Geometry check sheet. Reference: drawing and pictorial views, mm from the part's lowest x, y, z. A direction names the side the tool comes from. Round coordinates to 2 decimals unless told otherwise and drop trailing zeros. Write each loop counter-clockwise with the first axis right and the second up, starting at its lowest first coordinate (ties: lowest second). Pieces come first, ordered by that corner, then holes. Notation, with made-up numbers: M 74.25,16 L 122.25,16 A26 ccw 122.25,54 Z; hole C -5.5,69.25 d1. An arc over 180 degrees is marked long. Answer in a Markdown table with one row per item.
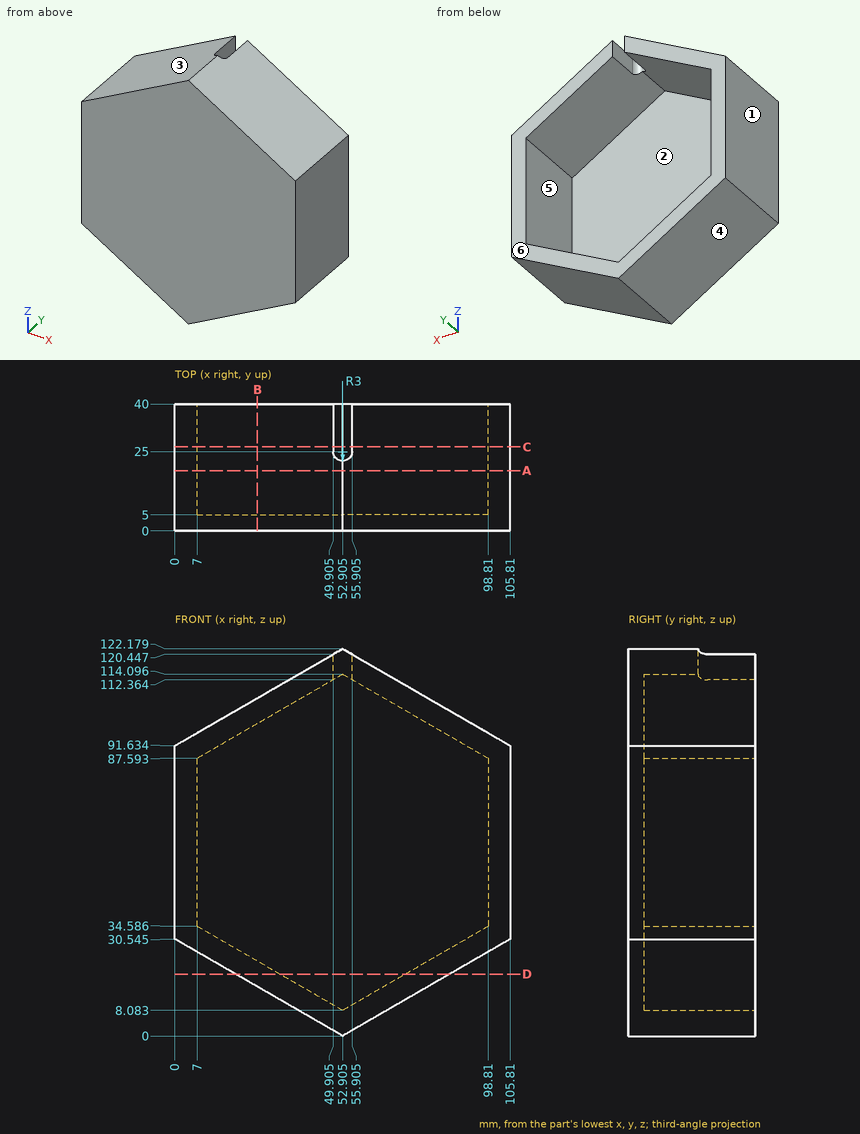
1. Access from +Z, -Z, +X, -X, +Y, -Y to the whole of each face (thin tool, end or side, straight path). Record for the marked faces 1 and 2.
Found:
| item | result |
|---|---|
| face 1 | +Z, -Z, -X, +Y, -Y |
| face 2 | +Y |
2. Section check A-A, the plane y = 19. Record the cut outline in (x, z) (1 decimal), and give its area (3 significant figures).
Found:
| item | result |
|---|---|
| outline | M 0,30.5 L 52.9,0 L 105.8,30.5 L 105.8,91.6 L 52.9,122.2 L 0,91.6 Z; hole M 7,34.6 L 52.9,8.1 L 98.8,34.6 L 98.8,87.6 L 52.9,114.1 L 7,87.6 Z |
| area | 2,400 mm2 |
3. Go/stop test with flat-tipped pins: pin 1 (12 mm diameter, centred on x = 45, z = 95.5, fed in from +Y); pin 2 (5 mm diameter, centred on x = 30, y = 22, fed in from +Z); pin 3 (10 mm diameter, centred on x = 18.5, y = 23.5, fed in from +Z). Record where each tip stops, or that it passes through.
Found:
| item | result |
|---|---|
| pin 1 | stops at y = 5 |
| pin 2 | stops at z = 110.4 |
| pin 3 | stops at z = 105.2 |
4. Draft check along Z on the marked faces 3, 4, 5 and 6. Enter one of: +Z half, -Z half, draft (parallel to the pull), parting line (faces both ways), or undercut.
Found:
| item | result |
|---|---|
| face 3 | +Z half |
| face 4 | -Z half |
| face 5 | undercut |
| face 6 | draft |
5. Section check C-C, the plane y = 26.5. Record the cut outline in (x, z) (1 decimal), and give its area (3 significant figures).
Found:
| item | result |
|---|---|
| outline | M 0,30.5 L 52.9,0 L 105.8,30.5 L 105.8,91.6 L 55.9,120.4 L 55.9,112.4 L 98.8,87.6 L 98.8,34.6 L 52.9,8.1 L 7,34.6 L 7,87.6 L 49.9,112.4 L 49.9,120.4 L 0,91.6 Z |
| area | 2,350 mm2 |
6. Scan lines: L1, parallel to X at y = 25.5, z = 62; L2, parallel to Y at x = 45, z = 69.5; L3, parallel to X at y = 26, z = 91.5 (1 decimal). Record each from-to range of solid material in increasing order.
Found:
| item | result |
|---|---|
| L1 | x = 0 to 7, 98.81 to 105.81 |
| L2 | y = 0 to 5 |
| L3 | x = 0 to 13.8, 92 to 105.8 |
7. Section check D-D, the plane z = 19.5. Record the cut outline in (x, y), and give its area (3 significant figures).
Found:
| item | result |
|---|---|
| outline | M 19.13,0 L 86.68,0 L 86.68,40 L 72.68,40 L 72.68,5 L 33.13,5 L 33.13,40 L 19.13,40 Z |
| area | 1,320 mm2 |
8. Section check B-B, the plane x = 26. Record the cut outline in (y, z) (1 decimal), and give its area (3 significant figures).
Found:
| item | result |
|---|---|
| outline | M 0,15.5 L 40,15.5 L 40,23.6 L 5,23.6 L 5,98.6 L 40,98.6 L 40,106.6 L 0,106.6 Z |
| area | 1,020 mm2 |
